Could you check a few things on this model? Use its own coordinates, in mm. A direction names the side the tool comes from. Round coordinates to 2 decimals unless told otherwise and drop trailing zeros. Write each loop counter-clockwise with the first axis right and the second up, starting at its lowest first coordinate (ties: lowest second). Pieces come first, ordered by that corner, then holes. Notation, with made-up numbers: (58.5, -5.5) - (93.5, -5.5) arc R30 cw to (93.5, 33.5) - close; hole circle Ø1 at (4, 83.25). An arc over 180 degrees is marked (long way). Write each question's results on one line, items separated by ' | '. Start each with the question number.
(1) For P1, Ø12, axis at x = -36, y = 18, coming from the -Z side; P2, Ø4, axis at x = 11.5, y = 7, coming from the -Z side; P3, Ø1.5, axis at x = -73.5, y = 26, coming from the +Z side, each with a flat end and sliding along its axis, tell me the tip position at first contact or that it passes through.
(2) Thinking about a two-plate mould opening in Z: for faces 4 (the cylindrical face through (43.985, 27.115, 1.161)), 5 (the flat face through (-95, 42, 0)), 6 (the flat face through (-86.653, 14, 0)), 7 (the flat face through (-56.389, 27.115, 27.942)), which applies, +Z half, -Z half, draft (parallel to the pull), parting line (faces both ways), or undercut?
(3) Imagine slicing it at D-D on z = -20. Write out the boundary of the cut face in (x, y), then the cut area to 3 significant figures.
(4) Imagine slicing it at A-A on z = 0. Write out the boundary of the cut face in (x, y), then the cut area to 3 significant figures.
(5) On a 3-axis mill with a long thin cutter (end or side, diameter ignored), from which of +Z, -Z, +X, -X, +Y, -Y can I reach the whole of each face in a straight line? I mean faces 1 (the flat face through (-48, 0, -29)), 2 (the flat face through (-74, 20, -15)), 3 (the flat face through (-77, 10, -10.35)). Say none if no direction works.
(6) Imagine slicing it at B-B on y = 50. Write out the boundary of the cut face in (x, z).
(7) Imagine slicing it at C-C on x = 0. Write out the boundary of the cut face in (y, z), then the cut area to 3 significant figures.
(8) Please list where these lines run through material, in increasing order: line 1 (X direction, y = 49.5, z = 1.5); line 2 (Z direction, x = 0, y = 40.5); line 3 (X direction, y = 17, z = 0). Write a range as [from, to].
```python
from build123d import *

# Parameters (mm, degrees)
BOSS_EXTRUDE1_DEPTH = 55
BOSS_EXTRUDE2_DEPTH = 28.5
BOSS_EXTRUDE3_DEPTH = 20


with BuildPart() as part:
    # Sketch1 → Boss-Extrude1 (new body)
    with BuildSketch(Plane(origin=(0, 0, 0), x_dir=(1, 0, 0), z_dir=(0, 1, 0))):
        with BuildLine():
            Line((-97.999995759, -14.422208071), (-13.596749299, -41.846487728))
            ThreePointArc((-13.596749299, -41.846487728), (44.00000144, 0), (-13.596749299, 41.846487728))
            Line((-13.596749299, 41.846487728), (-97.999995759, 14.422208071))
            Line((-97.999995759, 14.422208071), (-97.999995759, -14.422208071))
        make_face()
        with BuildLine():
            Line((-94.999995759, -12.242580547), (-12.669698241, -38.993318204))
            ThreePointArc((-12.669698241, -38.993318204), (41.00000144, 0), (-12.669698241, 38.993318204))
            Line((-12.669698241, 38.993318204), (-94.999995759, 12.242580547))
            Line((-94.999995759, 12.242580547), (-94.999995759, -12.242580547))
        make_face(mode=Mode.SUBTRACT)
    extrude(amount=BOSS_EXTRUDE1_DEPTH)

    # Sketch2 → Boss-Extrude2 (add)
    with BuildSketch(Plane.XZ):
        Polygon((-86.653035759, 14.954672498), (-86.653035759, -14.954672498), (-94.999995759, -12.242580547), (-94.999995759, 12.242580547), align=None)
    extrude(amount=-BOSS_EXTRUDE2_DEPTH)

    # Sketch3 → Boss-Extrude3 (add)
    with BuildSketch(Plane.XZ):
        Polygon((-86.653035759, -10.35), (-66.653035759, -10.35), (-66.653035759, -21.453067005), (-86.653035759, -14.954672498), align=None)
        Polygon((-66.653035759, 21.453067005), (-86.653035759, 14.954672498), (-86.653035759, 10.35), (-66.653035759, 10.35), align=None)
    extrude(amount=-BOSS_EXTRUDE3_DEPTH)


solid = part.part
```
Response:
1) P1: z = -36.52 | P2: z = -42.96 | P3: z = 22.63
2) face 4: parting line | face 5: undercut | face 6: undercut | face 7: +Z half
3) outline: (-80.83, 0) - (-66.65, 0) - (-66.65, 20) - (-71.13, 20) - (-71.13, 55) - (-80.83, 55) - close; (35.79, 0) - (39.19, 0) - (39.19, 55) - (35.79, 55) - close | area: 810 mm²
4) outline: (-98, 0) - (-86.65, 0) - (-86.65, 28.5) - (-95, 28.5) - (-95, 55) - (-98, 55) - close; (41, 0) - (44, 0) - (44, 55) - (41, 55) - close | area: 568 mm²
5) face 1: +Z, -Z, +X, -X, -Y | face 2: +Y | face 3: +Y, -Y
6) outline: (-98, -14.42) - (-13.6, -41.85) arc R44 ccw (long way) to (-13.6, 41.85) - (-98, 14.42) - close; hole (-95, -12.24) - (-12.67, -38.99) arc R41 ccw (long way) to (-12.67, 38.99) - (-95, 12.24) - close
7) outline: (0, -44) - (55, -44) - (55, -41) - (0, -41) - close; (0, 41) - (55, 41) - (55, 44) - (0, 44) - close | area: 330 mm²
8) line 1: [-98, -95], [40.97, 43.97] | line 2: [-44, -41], [41, 44] | line 3: [-98, -86.65], [41, 44]
